Read the model definition and answer for the solid it produces. Units are mm, in the model's axes. Face numbers are marked on the shaded views. A direction names the side the tool comes from. Coordinates: 2 decimals unless noted, no trailing zeros. Write each loop counter-clockwise with the first axis right and the second up, starting at its lowest first coordinate (ties: lowest second). Pieces come first, ordered by that corner, then holes.
(1) Find the intervals of material crossed by probe 1 along X at (y, z) = (-5.75, 23.75); probe 2 along Y at (x, z) = (-2.5, 20.5); probe 3 along X at (y, z) = (-7.5, 16), in increasing order.
(2) Which of the six approach directions +Z, -Z, +X, -X, +Y, -Y give full straight-line access (tool end or side, diameter ignored) to the marked faces 4 and 5?
(3) Given pin 1 (1.9 mm diameter, centred on x = -22, y = -8.5, fed in from +Z); pin 2 (8 mm diameter, centred on x = -16.5, y = 0, fed in from -Z), each flat-ended and moving along its own axis, determine where each tip first touches the part or whether it passes through.
(4) Section A-A on z = 16 is taken. Write down the section's boundary in (x, y) (3 decimals).
(5) Section B-B on y = -4.25 is taken. Write down the section's boundary in (x, z), then the cut area to 3 significant figures.
(6) Section C-C on x = -24.5 is taken. Write down the section's boundary in (y, z).
(7) The mould has two halves that part along Y. Classify the marked faces 1, 2 and 3: +Y half, -Y half, draft (parallel to the pull), parting line (faces both ways), or undercut.
from build123d import *

# Parameters (mm, degrees)
F0_W     = 37.465
F0_H     = 20.193
F1_DEPTH = 25.4
F3_DEPTH = 10.16
F4_R     = 2.54


with BuildPart() as f1:
    # F0 (on Top) → F1 (new body)
    with BuildSketch(Plane.XY):
        with Locations((-12.5743107353, -6.7907468112)):
            Rectangle(F0_W, F0_H)
    extrude(amount=F1_DEPTH)

    # F2 (on face) → F3 (cut)
    with BuildSketch(Plane.XY.offset(25.4)):
        with BuildLine():
            ThreePointArc((-25.5918107353, -6.7907468112), (-22.4168107353, -9.9657468112), (-19.2418107353, -6.7907468112))
            Line((-19.2418107353, -6.7907468112), (-25.5918107353, -6.7907468112))
        make_face()
        with BuildLine():
            Line((-25.5918107353, -6.7907468112), (-19.2418107353, -6.7907468112))
            ThreePointArc((-19.2418107353, -6.7907468112), (-22.4168107353, -3.6157468112), (-25.5918107353, -6.7907468112))
        make_face()
        with BuildLine():
            Line((-5.9068107353, -6.7907468112), (0.4431892647, -6.7907468112))
            ThreePointArc((0.4431892647, -6.7907468112), (-2.7318107353, -3.6157468112), (-5.9068107353, -6.7907468112))
        make_face()
        with BuildLine():
            ThreePointArc((-5.9068107353, -6.7907468112), (-2.7318107353, -9.9657468112), (0.4431892647, -6.7907468112))
            Line((0.4431892647, -6.7907468112), (-5.9068107353, -6.7907468112))
        make_face()
    extrude(amount=-F3_DEPTH, mode=Mode.SUBTRACT)

    # F4
    f4_edges = [f1.edges().sort_by_distance(p)[0] for p in [
        (-31.306811, -16.887247, 12.7),
        (6.158189, -16.887247, 12.7),
        (6.158189, 3.305753, 12.7),
        (-31.306811, 3.305753, 12.7),
    ]]
    fillet(f4_edges, radius=F4_R)


solid = f1.part
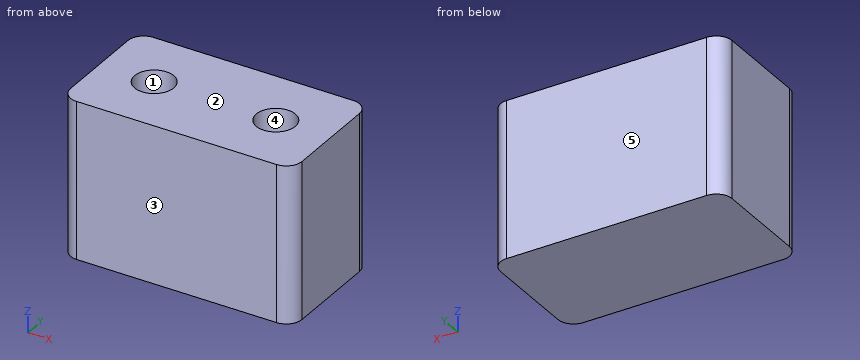
Response:
1. probe 1: x = -31.31 to -25.42, -19.42 to -5.73, 0.27 to 6.16
1. probe 2: y = -16.89 to -9.96, -3.62 to 3.31
1. probe 3: x = -31.31 to -25.51, -19.32 to -5.83, 0.36 to 6.16
2. face 4: +Z
2. face 5: +Z, -Z, +X, -X, +Y
3. pin 1: stops at z = 15.24
3. pin 2: stops at z = 0
4. outline: (-31.307, -14.347) arc R2.54 ccw to (-28.767, -16.887) - (3.618, -16.887) arc R2.54 ccw to (6.158, -14.347) - (6.158, 0.766) arc R2.54 ccw to (3.618, 3.306) - (-28.767, 3.306) arc R2.54 ccw to (-31.307, 0.766) - close; hole circle Ø6.35 at (-22.417, -6.791); hole circle Ø6.35 at (-2.732, -6.791)
5. outline: (-31.31, 0) - (6.16, 0) - (6.16, 25.4) - (-0.83, 25.4) - (-0.83, 15.24) - (-4.64, 15.24) - (-4.64, 25.4) - (-20.51, 25.4) - (-20.51, 15.24) - (-24.32, 15.24) - (-24.32, 25.4) - (-31.31, 25.4) - close
5. area: 874 mm2
6. outline: (-16.89, 0) - (3.31, 0) - (3.31, 25.4) - (-4.39, 25.4) - (-4.39, 15.24) - (-9.19, 15.24) - (-9.19, 25.4) - (-16.89, 25.4) - close
7. face 1: undercut
7. face 2: draft
7. face 3: -Y half
